Can you work these out from the model? Positions are in its coordinate system, mm. Give positions to 0.01 mm unless a question says otherwise; leave off trailing zeros. Write each loop counter-clockwise with the first axis right and the second up, starting at its lowest first coordinate (ties: lowest second). Pieces come first, ordered by that corner, then holes.
from build123d import *

# Parameters (mm, degrees)
F0_R      = 10
F1_DEPTH  = 25
F2_W      = 20
F2_H      = 24
F3_DEPTH  = 12.5
F4_SIZE   = 12.49999
F5_R      = 2
F9_R      = 3
F10_DEPTH = 25


# Not quite as in the source:
# - a fillet or chamfer is up to 0.001 mm smaller than in the source, because OpenCascade refuses the exact size


with BuildPart() as f1:
    # F0 (on Front) → F1 (new body)
    with BuildSketch(Plane.XZ):
        with BuildLine():
            ThreePointArc((-15, -5), (-12.0710678119, -12.0710678119), (-5, -15))
            Line((-5, -15), (5, -15))
            ThreePointArc((5, -15), (12.0710678119, -12.0710678119), (15, -5))
            Line((15, -5), (15, 15))
            Line((15, 15), (15, 445))
            Line((15, 445), (-15, 445))
            Line((-15, 445), (-15, 15))
            Line((-15, 15), (-15, -5))
        make_face()
        Circle(F0_R, mode=Mode.SUBTRACT)
    extrude(amount=F1_DEPTH)

    # F2 (on face) → F3 (cut)
    with BuildSketch(Plane(origin=(-15, 0, 0), x_dir=(0, -1, 0), z_dir=(-1, 0, 0))):
        with Locations((12.5, 410)):
            Rectangle(F2_W, F2_H)
    extrude(amount=-F3_DEPTH, mode=Mode.SUBTRACT)

    # F4 (size 12.5 in the source; OpenCascade refuses exactly that, so slightly less here)
    f4_edges = [f1.edges().sort_by_distance(p)[0] for p in [
        (-2.5, -12.5, 422),
    ]]
    chamfer(f4_edges, length=F4_SIZE)

    # F8: sweep along a path in F7
    with BuildLine(Plane.XY.offset(201)) as f8_path:
        ThreePointArc((-15, -18.75), (-21.25, -12.5), (-15, -6.25))
    # F5 (on face) → F8 (sweep)
    with BuildSketch(Plane(origin=(-15, 0, 0), x_dir=(0, -1, 0), z_dir=(-1, 0, 0))):
        with Locations((6.25, 201)):
            Circle(F5_R)
    sweep(path=f8_path.line)

    # F9 (on face) → F10 (cut, through all)
    with BuildSketch(Plane(origin=(0, 0, 0), x_dir=(-1, 0, 0), z_dir=(0, 1, 0))):
        with Locations((0, 372.5)):
            Circle(F9_R)
    extrude(amount=-F10_DEPTH, mode=Mode.SUBTRACT)


solid = f1.part
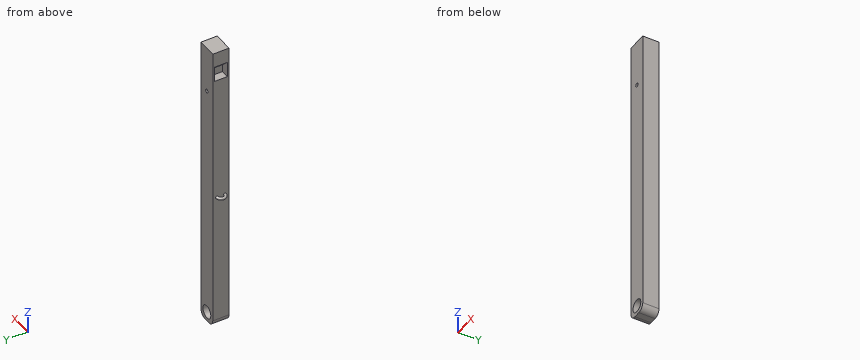
(1) Imagine slicing it at B-B, the plane z = 140. Write out the boundary of the cut face in (x, y).
Returned:
outline: (-15, -25) - (15, -25) - (15, 0) - (-15, 0) - close
(2) Will these pins go through, and if not, where does the flat tip stop? P1, Ø6.5, axis at x = -6.5, z = 406, coming from the +Y side; P2, Ø3, axis at y = -7, z = 311, coming from the -X side; P3, Ø16, axis at x = 0, z = 0, coming from the -Y side; P4, Ø3.5, axis at y = -10.5, z = 406.5, coming from the -X side.
Returned:
P1: stops at y = 0
P2: stops at x = -15
P3: passes through
P4: stops at x = -2.5
(3) Imagine slicing it at A-A, the plane z = 0. Write out the boundary of the cut face in (x, y).
Returned:
outline: (-15, -25) - (-10, -25) - (-10, 0) - (-15, 0) - close; (10, -25) - (15, -25) - (15, 0) - (10, 0) - close
(4) If I drill on L1, parallel to Z at x = 0, y = -8; L2, parallel to Z at x = -7, y = -16.25; L3, parallel to X at y = -10.5, z = 362.5, over which ranges is the centre line in solid material (lowest first)?
Returned:
L1: z = -15 to -10, 10 to 369.5, 375.5 to 445
L2: z = -14.8 to -7.14, 7.14 to 398, 414 to 445
L3: x = -15 to 15
